Design review of the part built by this model. Coordinates are the model's own, in mm. Give positions to 0.01 mm unless a question says otherwise; leave off trailing zeros. Loops run counter-clockwise (first coordinate to the right, second up) from the corner with the lowest first, then second, coordinate; pieces in that order, holes last. Notation, with made-up numbers: M -11.5,-1 L 3.5,-1 A24 ccw 3.5,17 Z; hole C 24,47.25 d8. An arc over 180 degrees is marked long. Use a Markdown table: item, result. Add a question column.
(1) Draft analysis for pull direction Z (two halves, no side actions). For faces 1 (the face through (0.55, 72.325, 82.074)), 2 (the face through (25, -12, 15)), 3 (the face through (-2.407, 72.325, 46.242)), state which applies: pulls with the +Z half, pulls with the -Z half, needs draft (parallel to the pull), parting line crosses it, or undercut.
(2) Add section D-D, the plane z = 50.5. Give the boundary of the cut face in (x, y), then the cut area to 3 significant figures.
(3) Insertion check: pin 1 Ø6 at (x, y) = (6.5, 16) entering from +Z; pin 2 Ø1.5 at (y, z) = (13.5, -34.5) entering from -X; pin 3 Ø10 at (x, y) = (-9.5, 73) entering from +Z. Each pin has a flat end and moves straight along its axis. Give the tip position at first contact, or say it passes through.
(4) For probe 1 along Z at (x, y) = (0, -12); probe 2 along Y at (x, z) = (-13, 1.5); probe 3 along Z at (x, y) = (0, 53), list the stretches that pass through material, from the lowest coordinate up.
(5) Add section B-B, the plane x = 0. Give the boundary of the cut face in (y, z).
(6) Add section A-A, the plane y = -9. Give the boundary of the cut face in (x, z).
(7) Add section C-C, the plane z = 70. Give the boundary of the cut face in (x, y).
```python
from build123d import *

# Parameters (mm, degrees)
F0_R     = 11.101292
F0_R_2   = 10.706517
F1_DEPTH = 25
F2_DEPTH = 30


with BuildPart() as f1:
    # F0 (on Front) → F1 (new body)
    with BuildSketch(Plane.XZ):
        with BuildLine():
            Line((-25, 57.079587), (-24.999876, -24.921242))
            ThreePointArc((-24.999876, -24.921242), (0.039379, -3.1e-05), (25, -25))
            Line((25, -25), (25, 57.079587))
            ThreePointArc((25, 57.079587), (0, 82.079587), (-25, 57.079587))
        make_face()
        with Locations((0, 57.079587)):
            Circle(F0_R, mode=Mode.SUBTRACT)
        with BuildLine():
            ThreePointArc((25, -25), (0.039379, -3.1e-05), (-24.999876, -24.921242))
            ThreePointArc((-24.999876, -24.921242), (-24.999969, -24.960621), (-25, -25))
            ThreePointArc((-25, -25), (0, -50), (25, -25))
        make_face()
        with Locations((0, -25)):
            Circle(F0_R_2, mode=Mode.SUBTRACT)
    extrude(amount=F1_DEPTH)

    # F0 (on Front) → F2 (join)
    with BuildSketch(Plane.XZ):
        with BuildLine():
            ThreePointArc((25, -25), (0.039379, -3.1e-05), (-24.999876, -24.921242))
            ThreePointArc((-24.999876, -24.921242), (-24.999969, -24.960621), (-25, -25))
            ThreePointArc((-25, -25), (0, -50), (25, -25))
        make_face()
        with Locations((0, -25)):
            Circle(F0_R_2, mode=Mode.SUBTRACT)
    extrude(amount=-F2_DEPTH)

    # F3: F1 across face


with BuildPart() as f1_1:
    add(f1.part)
    add(f1.part.mirror(Plane(origin=(0, 30, -25), x_dir=(1, 0, 0), z_dir=(0, 1, 0))))


solid = f1_1.part
```
Established:
| question | item | result |
|---|---|---|
| 1 | face 1 | pulls with the +Z half |
| 1 | face 2 | needs draft |
| 1 | face 3 | undercut |
| 2 | outline | M -25,-25 L -8.94,-25 L -8.94,0 L -25,0 Z; M -25,60 L -8.94,60 L -8.94,85 L -25,85 Z; M 8.94,-25 L 25,-25 L 25,0 L 8.94,0 Z; M 8.94,60 L 25,60 L 25,85 L 8.94,85 Z |
| 2 | area | 1,610 mm^2 |
| 3 | pin 1 | z = -0.25 |
| 3 | pin 2 | x = -23.42 |
| 3 | pin 3 | z = 81.67 |
| 4 | probe 1 | -50 to -35.71, -14.29 to 45.98, 68.18 to 82.08 |
| 4 | probe 2 | -25 to 0, 60 to 85 |
| 4 | probe 3 | -50 to -35.71, -14.29 to 0 |
| 5 | outline | M -25,-50 L 85,-50 L 85,-35.71 L -25,-35.71 Z; M -25,-14.29 L 85,-14.29 L 85,45.98 L 60,45.98 L 60,0 L 0,0 L 0,45.98 L -25,45.98 Z; M -25,68.18 L 0,68.18 L 0,82.08 L -25,82.08 Z; M 60,68.18 L 85,68.18 L 85,82.08 L 60,82.08 Z |
| 6 | outline | M -25,-25 A25 ccw 25,-25 L 25,57.08 A25 ccw -25,57.08 L -25,-24.92 A25.01 ccw Z; hole C 0,57.08 d22.2; hole C 0,-25 d21.41 |
| 7 | outline | M -21.4,-25 L 21.4,-25 L 21.4,0 L -21.4,0 Z; M -21.4,60 L 21.4,60 L 21.4,85 L -21.4,85 Z |
